from build123d import *

# Parameters (mm, degrees)
F0_R     = 18.15
F0_R_2   = 15.125
F1_DEPTH = 5
F2_R     = 23
F2_R_2   = 18.15
F2_R_3   = 15.125
F2_R_4   = 12.75
F3_DEPTH = 3
F4_R     = 15.75
F4_R_2   = 12.75
F5_DEPTH = 3


with BuildPart() as f1:
    # F0 (on Top) → F1 (new body)
    with BuildSketch(Plane.XY):
        Circle(F0_R)
        Circle(F0_R_2, mode=Mode.SUBTRACT)
    extrude(amount=F1_DEPTH)

    # F2 (on face) → F3 (join)
    with BuildSketch(Plane.XY.offset(5)):
        Circle(F2_R)
        Circle(F2_R_2, mode=Mode.SUBTRACT)
        Circle(F2_R_2)
        Circle(F2_R_3, mode=Mode.SUBTRACT)
        Circle(F2_R_3)
        Circle(F2_R_4, mode=Mode.SUBTRACT)
    extrude(amount=F3_DEPTH)

    # F4 (on face) → F5 (join)
    with BuildSketch(Plane.XY.offset(8)):
        Circle(F4_R)
        Circle(F4_R_2, mode=Mode.SUBTRACT)
    extrude(amount=F5_DEPTH)


solid = f1.part
Part model, mm, in its own coordinate system. A direction names the side the tool comes from. Round coordinates to 2 decimals unless told otherwise and drop trailing zeros. Order: outer loops, then holes, each group sorted by start corner. A loop starts at its lowest first (then second) coordinate and runs counter-clockwise, first axis right, second up. Notation, with made-up numbers: (83, 58.5) -> (93, 58.5) arc R26 ccw to (93, 77.5) -> close; hole circle Ø5 at (20.25, -36). An arc over 180 degrees is marked (long way). Put each result on its own line as item: value.
Q1. Band-saw the part on D-D (y = -13.5). Give the cut face in (x, z).
From the geometry:
outline: (-18.62, 5) -> (-12.13, 5) -> (-12.13, 0) -> (-6.82, 0) -> (-6.82, 5) -> (6.82, 5) -> (6.82, 0) -> (12.13, 0) -> (12.13, 5) -> (18.62, 5) -> (18.62, 8) -> (8.11, 8) -> (8.11, 11) -> (-8.11, 11) -> (-8.11, 8) -> (-18.62, 8) -> close
Q2. Pin check, flat tips, straight feed: pin 1 Ø23 at (x, y) = (0, 0) entering from -Z; pin 2 Ø12 at (x, y) = (-6.5, -3) entering from -Z; pin 3 Ø4 at (y, z) = (-17.5, 8) entering from -X; pin 4 Ø3 at (y, z) = (3.5, 6) entering from +X. Stop position of each tip, or through.
From the geometry:
pin 1: passes through
pin 2: stops at z = 5
pin 3: stops at x = -16.99
pin 4: stops at x = 22.91
Q3. Band-saw the part on B-B (y = 7). Give the cut face in (x, z).
From the geometry:
outline: (-21.91, 5) -> (-16.75, 5) -> (-16.75, 0) -> (-13.41, 0) -> (-13.41, 5) -> (-10.66, 5) -> (-10.66, 11) -> (-14.11, 11) -> (-14.11, 8) -> (-21.91, 8) -> close; (10.66, 5) -> (13.41, 5) -> (13.41, 0) -> (16.75, 0) -> (16.75, 5) -> (21.91, 5) -> (21.91, 8) -> (14.11, 8) -> (14.11, 11) -> (10.66, 11) -> close
Q4. Pull direction X, two halves, no side cores. Call faces 4 (the face through (-3.279, -14.765, 2.465)), 5 (the face through (-7, 14, 0)), 6 (the face through (17.312, 5.452, 2.465)): pulls with the +X half, pulls with the -X half, needs draft (parallel to the pull), parting line crosses it, or undercut.
From the geometry:
face 4: undercut
face 5: needs draft
face 6: parting line crosses it
Q5. Wall check: line 1 (Y direction, x = 0, z = 1.75) (3 decimals); line 2 (Y direction, x = 0, z = 7.5); line 3 (Z direction, x = 7, y = 21.5). Give the ranges that are in metal, low to high. Write a range as [from, to].
From the geometry:
line 1: y = [-18.15, -15.125], [15.125, 18.15]
line 2: y = [-23, -12.75], [12.75, 23]
line 3: z = [5, 8]
Q6. Band-saw the part on A-A (x = 0). Give the cut face in (y, z) (3 decimals), and give its area (3 significant figures).
From the geometry:
outline: (-23, 5) -> (-18.15, 5) -> (-18.15, 0) -> (-15.125, 0) -> (-15.125, 5) -> (-12.75, 5) -> (-12.75, 11) -> (-15.75, 11) -> (-15.75, 8) -> (-23, 8) -> close; (12.75, 5) -> (15.125, 5) -> (15.125, 0) -> (18.15, 0) -> (18.15, 5) -> (23, 5) -> (23, 8) -> (15.75, 8) -> (15.75, 11) -> (12.75, 11) -> close
area: 110 mm2
Q7. Band-saw the part on C-C (z = 1). Give the cut face in (x, y) (3 decimals), and give its area (3 significant figures).
From the geometry:
outline: circle Ø36.3 at (0, 0); hole circle Ø30.25 at (0, 0)
area: 316 mm2
Q8. Tool access for faces 1 (the face through (-2.994, 22.804, 6.479)), 2 (the face through (-2.05, 15.616, 9.479)), 3 (the face through (17, 7, 5)): list every direction of +Z, -Z, +X, -X, +Y, -Y with a clear straight run to the whole face (end or side of a thin tool).
From the geometry:
face 1: +Z, -Z
face 2: +Z
face 3: -Z
